For this review, take the finished solid that the model builds, in its own axes (mm). A direction names the side the tool comes from. Give positions to 0.01 mm unless a question says otherwise; leave off trailing zeros. Order: outer loops, then holes, each group sorted by start corner. A loop starts at its lowest first (then second) coordinate and runs counter-clockwise, first axis right, second up. Notation, with made-up numbers: (83.5, -12.5) - (136.5, -12.5) arc R26 cw to (136.5, 16.5) - close; hole circle Ø4 at (83.5, 56). An arc over 180 degrees is marked (long way). One line per item, written item: value.
```python
from build123d import *

# Parameters (mm, degrees)
EXTRUDE_1_DEPTH     = 60
SKETCH_4_R          = 4
CUT_EXTRUDE_3_DEPTH = 198


with BuildPart() as part:
    # 草图1 → 凸台-拉伸1 (new body)
    with BuildSketch(Plane.XY):
        Polygon((-100, 75), (100, 75), (100, 70), (60, 70), (60, -70), (100, -70), (100, -75), (-100, -75), (-100, -70), (-60, -70), (-60, 70), (-100, 70), align=None)
    extrude(amount=EXTRUDE_1_DEPTH)

    # 草图4 → 切除-拉伸3 (cut)
    with BuildSketch(Plane.XZ.offset(75)):
        with Locations(Location((-80, 30, 0), (0, 0, 270))):
            Circle(SKETCH_4_R)
        with Locations(Location((80, 30, 0), (0, 0, 270))):
            Circle(SKETCH_4_R)
    extrude(amount=-CUT_EXTRUDE_3_DEPTH, mode=Mode.SUBTRACT)


solid = part.part
```
(1) Machinability: for faces 1 (the face through (75, -70, 30)), 2 (the face through (-85, -70, 30)), 3 (the face through (-83.905, -72.535, 30.867)), which of the approach directions +Z, -Z, +X, -X, +Y, -Y give a long, thin tool a straight path to every point of the face, cutting with its end or side? Answer none if there is none.
Answers below:
face 1: +Z, -Z, +X
face 2: +Z, -Z, -X
face 3: +Y, -Y
(2) For P1, Ø9, axis at x = 80, z = 30, coming from the -Y side; P2, Ø1.5, axis at x = -62.5, y = 13, coming from the +Z side; P3, Ø12, axis at y = -58.5, z = 49.5, coming from the +X side; P4, Ø12, axis at y = -1, z = 27.5, coming from the -X side, all flat-tipped, find the tip position at first contact; note any pin that passes through.
Answers below:
P1: stops at y = -75
P2: passes through
P3: stops at x = 60
P4: stops at x = -60
(3) Take a section at C-C (z = 14.5). Write out the cut boundary in (x, y), then the cut area to 3 significant figures.
Answers below:
outline: (-100, -75) - (100, -75) - (100, -70) - (60, -70) - (60, 70) - (100, 70) - (100, 75) - (-100, 75) - (-100, 70) - (-60, 70) - (-60, -70) - (-100, -70) - close
area: 18,800 mm^2
(4) Draft analysis for pull direction Y (two halves, no side actions). For faces 4 (the face through (60, 1, 30)), 5 (the face through (1, -75, 30)), 6 (the face through (100, -72, 30)), state which applies: pulls with the +Y half, pulls with the -Y half, needs draft (parallel to the pull), parting line crosses it, or undercut.
Answers below:
face 4: undercut
face 5: pulls with the -Y half
face 6: needs draft
(5) Take a section at B-B (x = -80). Write out the cut boundary in (y, z), then the cut area to 3 significant figures.
Answers below:
outline: (-75, 0) - (-70, 0) - (-70, 26) - (-75, 26) - close; (-75, 34) - (-70, 34) - (-70, 60) - (-75, 60) - close; (70, 0) - (75, 0) - (75, 26) - (70, 26) - close; (70, 34) - (75, 34) - (75, 60) - (70, 60) - close
area: 520 mm^2
(6) Wall thickness on line 1 (X direction, y = -72, z = 30); line 2 (Y direction, x = 65.5, z = 23.5); line 3 (X direction, y = -44, z = 38): over which ranges is each line inside the solid? List them lowest first. Write a range as from..to.
Answers below:
line 1: x = -100..-84, -76..76, 84..100
line 2: y = -75..-70, 70..75
line 3: x = -60..60
(7) Take a section at A-A (z = 30). Write out the cut boundary in (x, y), then the cut area to 3 significant figures.
Answers below:
outline: (-100, -75) - (-84, -75) - (-84, -70) - (-100, -70) - close; (-100, 70) - (-84, 70) - (-84, 75) - (-100, 75) - close; (-76, -75) - (76, -75) - (76, -70) - (60, -70) - (60, 70) - (76, 70) - (76, 75) - (-76, 75) - (-76, 70) - (-60, 70) - (-60, -70) - (-76, -70) - close; (84, -75) - (100, -75) - (100, -70) - (84, -70) - close; (84, 70) - (100, 70) - (100, 75) - (84, 75) - close
area: 18,600 mm^2
(8) Take a section at D-D (y = -16.5). Write out the cut boundary in (x, z).
Answers below:
outline: (-60, 0) - (60, 0) - (60, 60) - (-60, 60) - close
